```python
from build123d import *

# Parameters (mm, degrees)
F0_R      = 12
F1_DEPTH  = 64
F2_R      = 13.5
F3_DEPTH  = 8
F5_DEPTH  = 7.5
F7_DEPTH  = 12.5
F10_R     = 8
F11_DEPTH = 24.001
F12_R     = 2
F13_R     = 8
F14_DEPTH = 28
F16_DEPTH = 8


with BuildPart() as f1:
    # F0 (on Top) → F1 (new body)
    with BuildSketch(Plane.XY):
        Circle(F0_R)
    extrude(amount=F1_DEPTH)

    # F2 (on Top) → F3 (join)
    with BuildSketch(Plane.XY):
        Circle(F2_R)
    extrude(amount=F3_DEPTH)

    # F4 (on Front) → F5 (join, symmetric)
    with BuildSketch(Plane.XZ):
        with BuildLine():
            Line((12, 40), (19.042305, 55.146153))
            ThreePointArc((19.042305, 55.146153), (0, 85), (-19.042305, 55.146153))
            Line((-19.042305, 55.146153), (-12, 40))
            Line((-12, 40), (12, 40))
        make_face()
    extrude(amount=F5_DEPTH, both=True)

    # F6 (on Right) → F7 (cut, symmetric)
    with BuildSketch(Plane.YZ):
        Polygon((-7.5, 40), (-7.5, 64), (-12, 64), (-12, 35.5), align=None)
        Polygon((12, 64), (7.5, 64), (7.5, 40), (12, 35.5), align=None)
    extrude(amount=F7_DEPTH, both=True, mode=Mode.SUBTRACT)

    # F8 (on Right) → F9 (revolve)
    with BuildSketch(Plane.YZ):
        Polygon((-10.5, 74), (-10.5, 64), (10.5, 64), (10.5, 74.892095), (7.5, 76), (-7.5, 76), align=None)
    revolve(axis=Axis((0, 1.309478, 64), (0, 1, 0)))

    # F10 (on face) → F11 (cut, through all)
    with BuildSketch(Plane.XZ.offset(10.5)):
        with Locations((0, 64)):
            Circle(F10_R)
    extrude(amount=-F11_DEPTH, mode=Mode.SUBTRACT)

    # F12
    f12_edges = [f1.edges().sort_by_distance(p)[0] for p in [
        (15.521153, -7.5, 47.573076),
        (15.521153, 7.5, 47.573076),
    ]]
    fillet(f12_edges, radius=F12_R)

    # F13 (on face) → F14 (cut)
    with BuildSketch(Plane(origin=(0, 0, 0), x_dir=(1, 0, 0), z_dir=(0, 0, -1))):
        Circle(F13_R)
    extrude(amount=-F14_DEPTH, mode=Mode.SUBTRACT)

    # F15 (on face) → F16 (cut, through all)
    with BuildSketch(Plane(origin=(0, 0, 0), x_dir=(1, 0, 0), z_dir=(0, 0, -1))):
        with BuildLine():
            Line((-11, -7.826238), (-11, 7.826238))
            ThreePointArc((-11, 7.826238), (-13.5, 0), (-11, -7.826238))
        make_face()
        with BuildLine():
            Line((11, 7.826238), (11, -7.826238))
            ThreePointArc((11, -7.826238), (13.5, 0), (11, 7.826238))
        make_face()
    extrude(amount=-F16_DEPTH, mode=Mode.SUBTRACT)


solid = f1.part
```
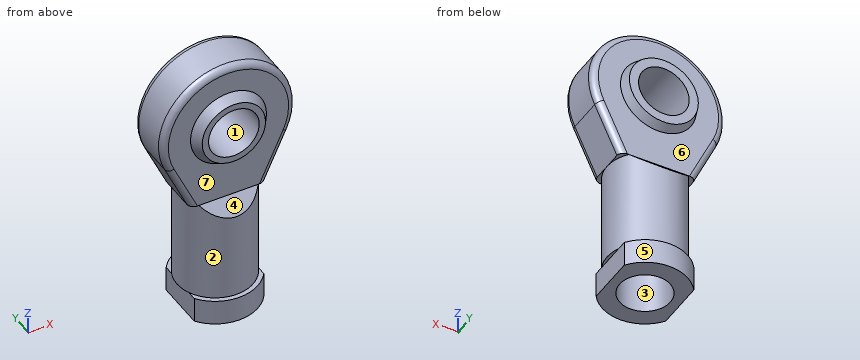
The model under review builds one solid part; all positions refer to its coordinate system, in mm. Face numbers are marked on the shaded views. A direction names the side the tool comes from. Give positions to 0.01 mm unless a question says otherwise; leave off trailing zeros. Loops run counter-clockwise (first coordinate to the right, second up) from the corner with the lowest first, then second, coordinate; pieces in that order, holes last. Notation, with made-up numbers: (47.25, 81.5) - (92.25, 81.5) arc R25 cw to (92.25, 119.5) - close; hole circle Ø11 at (6, 54.25). An arc over 180 degrees is marked (long way). Answer as a JSON object with one key per item and string values.
Q1. Add section D-D on y = -3.75. State the section outline as (x, z) points.
Worked out:
{"outline": "(-19.04, 55.15) - (-12, 40) - (-11.4, 40) - (-11.4, 8) - (-11, 8) - (-11, 0) - (-7.07, 0) - (-7.07, 28) - (7.07, 28) - (7.07, 0) - (11, 0) - (11, 8) - (11.4, 8) - (11.4, 40) - (12, 40) - (19.04, 55.15) arc R21 ccw (long way) to start; hole circle Ø16 at (0, 64)"}
Q2. To check wall thickness, follow line 1 along X through (y, z) = (0, 9.5); line 2 along Z through (x, y) = (2, -8); line 3 along Z through (x, y) = (-6.5, 1.75). State the ranges of each line that lie inside material, in increasing order.
Worked out:
{"line 1": "x = -12 to -8, 8 to 12", "line 2": "z = 0 to 39.5, 52.51 to 56.25, 71.75 to 75.49", "line 3": "z = 28 to 59.34, 68.66 to 83.97"}
Q3. For the marked faces 5, 6 and 7, list the 3-axis set-ups (+Z, -Z, +X, -X, +Y, -Y) from which the entire face can be reached by the end or side of a thin tool; tool diameter is ignored.
Worked out:
{"face 5": "-Z, +Y", "face 6": "+Y", "face 7": "-Y"}
Q4. Mouldability with a two-part tool opening along Y and no side actions: class the marked faces 1, 2, 3 and 4 as +Y half, -Y half, draft (parallel to the pull), parting line (faces both ways), or undercut.
Worked out:
{"face 1": "draft", "face 2": "parting line", "face 3": "undercut", "face 4": "-Y half"}
Q5. Add section C-C on z = 9.5. State the section outline as (x, y) points, plus the area to 3 significant figures.
Worked out:
{"outline": "circle Ø24 at (0, 0); hole circle Ø16 at (0, 0)", "area": "251 mm^2"}
Q6. Add section B-B on y = 1.75. State the section outline as (x, z) points, plus the area to 3 significant figures.
Worked out:
{"outline": "(-19.04, 55.15) - (-12, 40) - (-11.87, 40) - (-11.87, 8) - (-11, 8) - (-11, 0) - (-7.81, 0) - (-7.81, 28) - (7.81, 28) - (7.81, 0) - (11, 0) - (11, 8) - (11.87, 8) - (11.87, 40) - (12, 40) - (19.04, 55.15) arc R21 ccw (long way) to start; hole circle Ø16 at (0, 64)", "area": "1,820 mm^2"}
Q7. Insertion check: pin 1 (4 mm diameter, centred on y = -1, z = 3.5, fed in from +X); pin 2 (2 mm diameter, centred on x = -1.5, z = 36, fed in from -Y); pin 3 (1 mm diameter, centred on x = 3.5, y = -0.5, fed in from +Z). Each pin has a flat end and moves straight along its axis. Give the tip position at first contact, or say it passes through.
Worked out:
{"pin 1": "stops at x = 11", "pin 2": "stops at y = -11.98", "pin 3": "stops at z = 84.78"}
